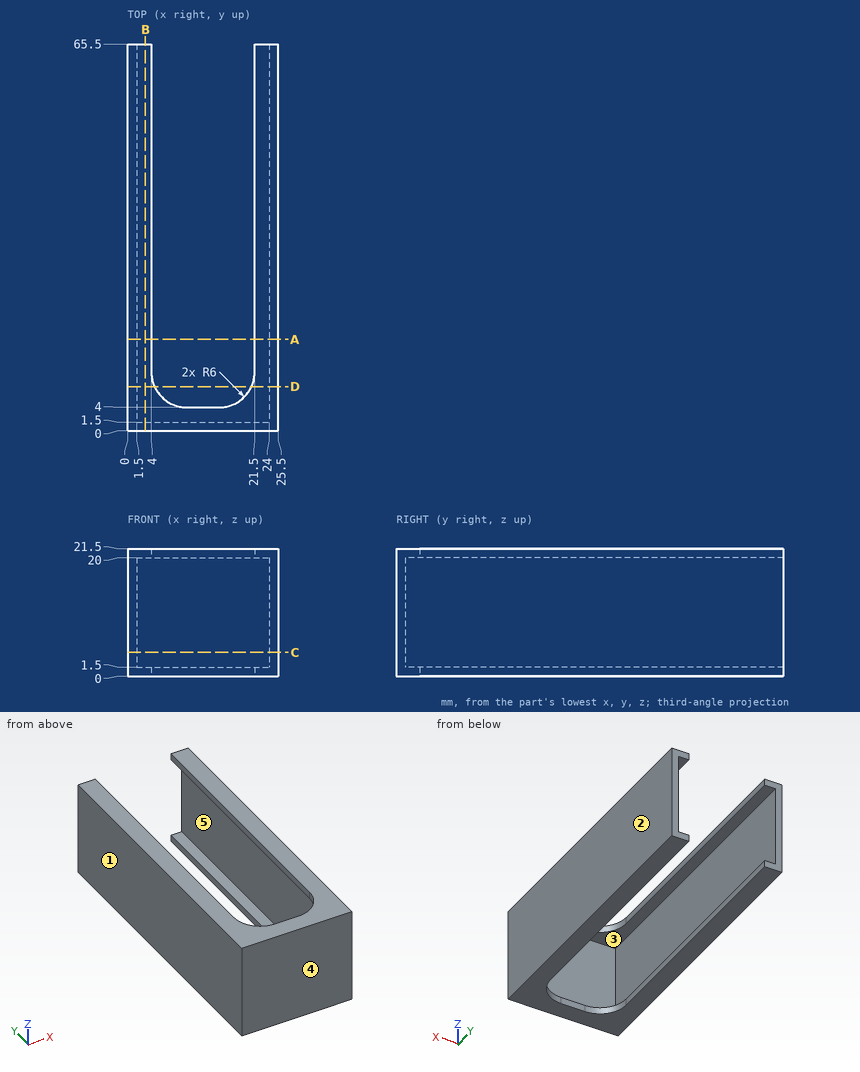
Geometry: see drawing. Coordinates: mm, zero at the bounding-box minimum. A direction names the side the tool comes from. Give positions to 0.01 mm unless a question says otherwise; leave off trailing zeros. Write each loop counter-clockwise with the first axis right and the second up, starting at its lowest first coordinate (ties: lowest second). Pieces come first, ordered by that corner, then holes. Notation, with made-up numbers: M 88,-11.5 L 122,-11.5 A22 cw 122,20.5 Z; hole C 13.25,12 d4. An arc over 180 degrees is marked long. Answer as a JSON object with one key per item and string values.
Q1. Contact query for flat-ended pins moving along their axis: P1, Ø1.2, axis at x = 12, z = 21, coming from the +Y side; P2, Ø2, axis at x = 19.5, z = 13.5, coming from the +Y side. Output: stop coordinate, or through.
Geometry check:
{"P1": "stops at y = 4", "P2": "stops at y = 1.5"}
Q2. Cut plane A-A, the plane y = 15.5. Return the cut outline in (x, z), then the cut area to 3 significant figures.
Geometry check:
{"outline": "M 0,0 L 4,0 L 4,1.5 L 1.5,1.5 L 1.5,20 L 4,20 L 4,21.5 L 0,21.5 Z; M 21.5,0 L 25.5,0 L 25.5,21.5 L 21.5,21.5 L 21.5,20 L 24,20 L 24,1.5 L 21.5,1.5 Z", "area": "79.5 mm^2"}
Q3. Access query for the marked faces 4 and 5. Directions: +Z, -Z, +X, -X, +Y, -Y. A direction counts if a zero-diameter tool reaches every point of the face in a straight line with its end or side. Return the directions, or none.
Geometry check:
{"face 4": "+Z, -Z, +X, -X, -Y", "face 5": "+Y"}
Q4. Cut plane D-D, the plane y = 7.5. Return the cut outline in (x, z), then the cut area to 3 significant figures.
Geometry check:
{"outline": "M 0,0 L 4.55,0 L 4.55,1.5 L 1.5,1.5 L 1.5,20 L 4.55,20 L 4.55,21.5 L 0,21.5 Z; M 20.95,0 L 25.5,0 L 25.5,21.5 L 20.95,21.5 L 20.95,20 L 24,20 L 24,1.5 L 20.95,1.5 Z", "area": "82.8 mm^2"}
Q5. Mould query, pull axis X, two halves, no side actions, for the marked faces 1, 2 and 3. Classes: +X half, -X half, draft (parallel to the pull), parting line (faces both ways), or undercut.
Geometry check:
{"face 1": "-X half", "face 2": "+X half", "face 3": "undercut"}
Q6. Ray query, line 1 along X through (y, z) = (35, 2.75); line 2 along Z through (x, y) = (22.75, 14); line 3 along Y through (x, z) = (21.5, 12.75). Return the intervals inside material, ascending.
Geometry check:
{"line 1": "x = 0 to 1.5, 24 to 25.5", "line 2": "z = 0 to 1.5, 20 to 21.5", "line 3": "y = 0 to 1.5"}
Q7. Cut plane B-B, the plane x = 3. Return the cut outline in (y, z).
Geometry check:
{"outline": "M 0,0 L 65.5,0 L 65.5,1.5 L 1.5,1.5 L 1.5,20 L 65.5,20 L 65.5,21.5 L 0,21.5 Z"}
Q8. Cut plane C-C, the plane z = 4. Return the cut outline in (x, y).
Geometry check:
{"outline": "M 0,0 L 25.5,0 L 25.5,65.5 L 24,65.5 L 24,1.5 L 1.5,1.5 L 1.5,65.5 L 0,65.5 Z"}
